Model file for the job. Use its own axes, mm. Face numbers are marked on the shaded views. A direction names the side the tool comes from. Round coordinates to 2 decimals unless told otherwise and drop trailing zeros. Loops run counter-clockwise (first coordinate to the right, second up) from the corner with the lowest first, then second, coordinate; pieces in that order, holes last.
from build123d import *

# Parameters (mm, degrees)
SKETCH1_W            = 66.35
SKETCH1_H            = 69.18
BOSS_EXTRUDE1_DEPTH  = 2
SKETCH2_R            = 31
CUT_EXTRUDE1_DEPTH   = 48.969247701
M3_CLEARANCE_HOLE1_D = 3.2
BOSS_EXTRUDE2_START  = -3
SKETCH6_R            = 32
SKETCH6_R_2          = 31
BOSS_EXTRUDE2_DEPTH  = 3
FILLET1_R            = 1


with BuildPart() as part:
    # Sketch1 → Boss-Extrude1 (new body)
    with BuildSketch(Plane(origin=(0, 0, 0), x_dir=(0, 0, -1), z_dir=(1, 0, 0))):
        Rectangle(SKETCH1_W, SKETCH1_H)
    extrude(amount=BOSS_EXTRUDE1_DEPTH)

    # Sketch2 → Cut-Extrude1 (cut, through all)
    with BuildSketch(Plane.ZY):
        with Locations((0, 1.91)):
            Circle(SKETCH2_R)
    extrude(amount=-CUT_EXTRUDE1_DEPTH, mode=Mode.SUBTRACT)

    # M3 Clearance Hole1 (through all)
    with Locations(Plane(origin=(2, 0, 0), x_dir=(0, 0, -1), z_dir=(1, 0, 0))):
        with Locations((-22.5, 29.91), (22.5, -26.09)):
            Hole(M3_CLEARANCE_HOLE1_D / 2)

    # Sketch6 → Boss-Extrude2 (add)
    with BuildSketch(Plane(origin=(0, 0, 0), x_dir=(0, 0, -1), z_dir=(1, 0, 0)).offset(BOSS_EXTRUDE2_START)):
        with Locations((0, 1.91)):
            Circle(SKETCH6_R)
        with Locations(Location((0, 1.91, 0), (0, 0, 180))):
            Circle(SKETCH6_R_2, mode=Mode.SUBTRACT)
    extrude(amount=BOSS_EXTRUDE2_DEPTH)

    # Fillet1
    fillet1_edges = [part.edges().sort_by_distance(p)[0] for p in [
        (1, -34.59, -33.175),
        (1, -34.59, 33.175),
        (1, 34.59, 33.175),
        (1, 34.59, -33.175),
    ]]
    fillet(fillet1_edges, radius=FILLET1_R)


solid = part.part
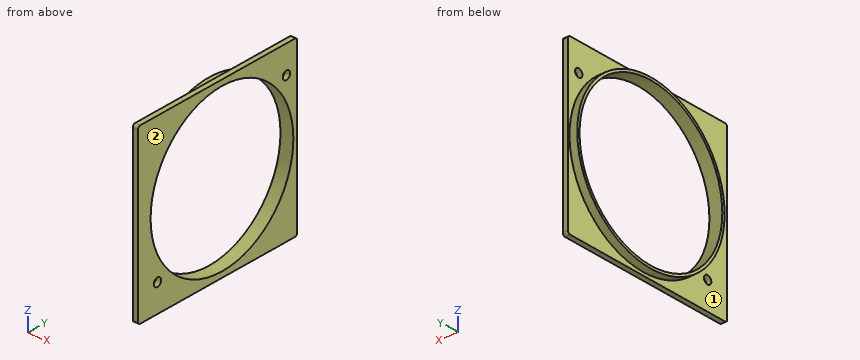
Q1. Slice it at D-D on z = -22.5. Give the cut face in (x, y).
Q2. Slice it at C-C on z = 0. Give the cut face in (x, y), plus the area to 3 significant figures.
Q3. Probe line 1 (Y direction, x = 1.1, z = -22.5); line 2 (Y direction, x = 0.5, z = 0); line 3 (Y direction, x = 1.55, z = 22.5). List the from-to ranges inside material, lowest first.
Q4. Slice it at A-A on y = 1.91. Give the cut face in (x, z) (3 decimals).
Q5. Tool access for the marked faces 1 and 2: list every direction of +Z, -Z, +X, -X, +Y, -Y with a clear straight run to the whole face (end or side of a thin tool).
Q6. Flat gauge pins, fed straight in: P1, Ø1.9, axis at y = 29.91, z = 22.5, coming from the -X side; P2, Ø1.5, axis at x = -1.5, z = -19, coming from the -Y side. Where does each tip first touch, or does it go through?
Q7. Slice it at B-B on x = 1.25. Give the cut face in (y, z) (3 decimals), plus the area to 3 significant figures.
Reply:
1. outline: (-3, -20.84) - (0, -20.84) - (0, -24.49) - (2, -24.49) - (2, -19.41) - (-3, -19.41) - close; (-3, 23.23) - (2, 23.23) - (2, 34.59) - (0, 34.59) - (0, 24.66) - (-3, 24.66) - close; (0, -34.59) - (2, -34.59) - (2, -27.69) - (0, -27.69) - close
2. outline: (-3, -30.09) - (0, -30.09) - (0, -34.59) - (2, -34.59) - (2, -29.09) - (-3, -29.09) - close; (-3, 32.91) - (2, 32.91) - (2, 34.59) - (0, 34.59) - (0, 33.91) - (-3, 33.91) - close
2. area: 20.4 mm2
3. line 1: y = -34.59 to -27.69, -24.49 to -19.41, 23.23 to 34.59
3. line 2: y = -34.59 to -29.09, 32.91 to 34.59
3. line 3: y = -34.59 to -19.41, 23.23 to 28.31, 31.51 to 34.59
4. outline: (-3, -32) - (0, -32) - (0, -33.175) - (2, -33.175) - (2, -31) - (-3, -31) - close; (-3, 31) - (2, 31) - (2, 33.175) - (0, 33.175) - (0, 32) - (-3, 32) - close
5. face 1: -X
5. face 2: +Z, -Z, +X, +Y, -Y
6. P1: passes through
6. P2: stops at y = -24.38
7. outline: (-34.59, -32.175) arc R1 ccw to (-33.59, -33.175) - (33.59, -33.175) arc R1 ccw to (34.59, -32.175) - (34.59, 32.175) arc R1 ccw to (33.59, 33.175) - (-33.59, 33.175) arc R1 ccw to (-34.59, 32.175) - close; hole circle Ø62 at (1.91, 0); hole circle Ø3.2 at (-26.09, -22.5); hole circle Ø3.2 at (29.91, 22.5)
7. area: 1,550 mm2
